```python
from build123d import *

# Parameters (mm, degrees)
F0_W     = 98
F0_H     = 68
F0_R     = 2.1
F1_DEPTH = 35
F2_W     = 90
F2_H     = 60
F3_DEPTH = 4
F4_R     = 5
F5_R     = 5


with BuildPart() as f1:
    # F0 (on Top) → F1 (new body)
    with BuildSketch(Plane.XY):
        Rectangle(F0_W, F0_H)
        with Locations((-41, -26)):
            Circle(F0_R, mode=Mode.SUBTRACT)
        with Locations((41, -26)):
            Circle(F0_R, mode=Mode.SUBTRACT)
        with BuildLine():
            ThreePointArc((45, -26), (38.171573, -23.171573), (41, -30))
            Line((41, -30), (-41, -30))
            ThreePointArc((-41, -30), (-38.171573, -23.171573), (-45, -26))
            Line((-45, -26), (-45, 26))
            ThreePointArc((-45, 26), (-38.171573, 23.171573), (-41, 30))
            Line((-41, 30), (41, 30))
            ThreePointArc((41, 30), (38.171573, 23.171573), (45, 26))
            Line((45, 26), (45, -26))
        make_face(mode=Mode.SUBTRACT)
        with Locations((-41, 26)):
            Circle(F0_R, mode=Mode.SUBTRACT)
        with Locations((41, 26)):
            Circle(F0_R, mode=Mode.SUBTRACT)
    extrude(amount=F1_DEPTH)

    # F2 (on Top) + F0 (on Top) → F3 (join)
    with BuildSketch(Plane.XY):
        Rectangle(F2_W, F2_H)
    with BuildSketch(Plane.XY):
        Rectangle(F0_W, F0_H)
        with Locations((-41, -26)):
            Circle(F0_R, mode=Mode.SUBTRACT)
        with Locations((41, -26)):
            Circle(F0_R, mode=Mode.SUBTRACT)
        with BuildLine():
            ThreePointArc((45, -26), (38.171573, -23.171573), (41, -30))
            Line((41, -30), (-41, -30))
            ThreePointArc((-41, -30), (-38.171573, -23.171573), (-45, -26))
            Line((-45, -26), (-45, 26))
            ThreePointArc((-45, 26), (-38.171573, 23.171573), (-41, 30))
            Line((-41, 30), (41, 30))
            ThreePointArc((41, 30), (38.171573, 23.171573), (45, 26))
            Line((45, 26), (45, -26))
        make_face(mode=Mode.SUBTRACT)
        with Locations((-41, 26)):
            Circle(F0_R, mode=Mode.SUBTRACT)
        with Locations((41, 26)):
            Circle(F0_R, mode=Mode.SUBTRACT)
    extrude(amount=F3_DEPTH)

    # F4
    f4_edges = [f1.edges().sort_by_distance(p)[0] for p in [
        (49, -34, 17.5),
        (-49, -34, 17.5),
        (-49, 34, 17.5),
    ]]
    fillet(f4_edges, radius=F4_R)

    # F5
    f5_edges = [f1.edges().sort_by_distance(p)[0] for p in [
        (49, 34, 17.5),
        (2.5, 34, 0),
    ]]
    fillet(f5_edges, radius=F5_R)


solid = f1.part
```
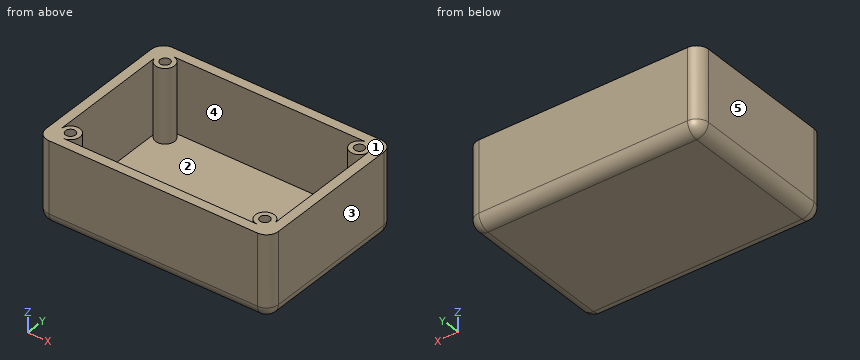
Can you work these out from the model? Positions are in its coordinate system, mm. Face numbers are marked on the shaded views. A direction names the side the tool comes from. Coordinates: 2 decimals unless noted, no trailing zeros. Order: outer loops, then holes, each group sorted by start corner. A loop starts at its lowest first (then second) coordinate and runs counter-clockwise, first axis right, second up. Notation, with made-up numbers: (-10.75, 50.5) - (42.25, 50.5) arc R12 cw to (42.25, 68.5) - close; hole circle Ø11 at (18.5, 80). An arc over 180 degrees is marked (long way). Answer in a Markdown table with one row per item.
1. If I drill on line 1 along Y through (x, z) = (1, 30); line 2 along X through (y, z) = (-1, 7); line 3 along Y through (x, z) = (41.5, 15), over which ranges is the centre line in solid material (lowest first)?
Reply:
| item | result |
|---|---|
| line 1 | y = -34 to -30, 30 to 34 |
| line 2 | x = -49 to -45, 45 to 49 |
| line 3 | y = -34 to -28.04, -23.96 to -22.03, 22.03 to 23.96, 28.04 to 34 |
2. For the marked faces 1 and 2, which set-ups out of +Z, -Z, +X, -X, +Y, -Y let a thin tool reach every point of the face, with its end or its side?
Reply:
| item | result |
|---|---|
| face 1 | +Z, +X, -X, +Y, -Y |
| face 2 | +Z |
3. Suppose I cut it at B-B (x = -21). Please give me the cut outline in (y, z).
Reply:
| item | result |
|---|---|
| outline | (-34, 5) arc R5 ccw to (-29, 0) - (29, 0) arc R5 ccw to (34, 5) - (34, 35) - (30, 35) - (30, 4) - (-30, 4) - (-30, 35) - (-34, 35) - close |
4. Suppose I cut it at C-C (y = 20). Please give me the cut outline in (x, z), and give its area (3 significant figures).
Reply:
| item | result |
|---|---|
| outline | (-49, 5) arc R5 ccw to (-44, 0) - (44, 0) arc R5 ccw to (49, 5) - (49, 35) - (45, 35) - (45, 4) - (-45, 4) - (-45, 35) - (-49, 35) - close |
| area | 629 mm^2 |
5. If we mould it in two halves opening along X, with no side actions, what happens to the marked faces 3, 4 and 5? For each: pulls with the +X half, pulls with the -X half, needs draft (parallel to the pull), parting line crosses it, or undercut.
Reply:
| item | result |
|---|---|
| face 3 | pulls with the +X half |
| face 4 | undercut |
| face 5 | pulls with the -X half |
6. Suppose I cut it at A-A (z = 26). Please give me the cut outline in (x, y).
Reply:
| item | result |
|---|---|
| outline | (-49, -29) arc R5 ccw to (-44, -34) - (44, -34) arc R5 ccw to (49, -29) - (49, 29) arc R5 ccw to (44, 34) - (-44, 34) arc R5 ccw to (-49, 29) - close; hole (-45, -26) arc R4 cw (long way) to (-41, -30) - (41, -30) arc R4 cw (long way) to (45, -26) - (45, 26) arc R4 cw (long way) to (41, 30) - (-41, 30) arc R4 cw (long way) to (-45, 26) - close; hole circle Ø4.2 at (-41, -26); hole circle Ø4.2 at (-41, 26); hole circle Ø4.2 at (41, -26); hole circle Ø4.2 at (41, 26) |
7. For pin 1 (12 mm diameter, centred on x = 9, y = -18.5, fed in from +Z), with a flat end and sliding along its axis, tell me the tip position at first contact or that it passes through.
Reply:
| item | result |
|---|---|
| pin 1 | stops at z = 4 |
